Verification items for the finished model (mm, model axes). Round coordinates to 2 decimals unless told otherwise and drop trailing zeros. Loops run counter-clockwise (first coordinate to the right, second up) from the corner with the lowest first, then second, coordinate; pieces in that order, holes last. Notation, with made-up numbers: (1, 19.25) -> (22, 19.25) arc R16 ccw to (22, 33.25) -> close; hole circle Ø6 at (80, -36.75). An arc over 180 degrees is marked (long way). Write item = value, one per line.
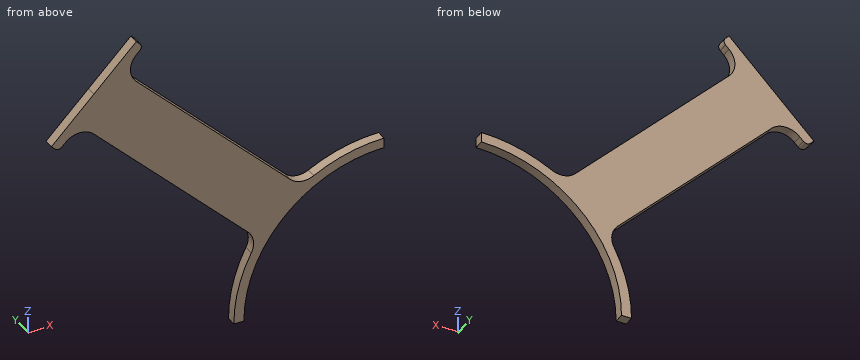
```python
from build123d import *

# Parameters (mm, degrees)
BOSS_EXTRUDE1_DEPTH = 5
FILLET1_R           = 10
FILLET2_R           = 2.5


with BuildPart() as part:
    # Sketch2 → Boss-Extrude1 (new body)
    with BuildSketch(Plane(origin=(0, 0, 0), x_dir=(1, 0, 0), z_dir=(0, 1, 0))):
        with BuildLine():
            Line((-70, 0), (-75, 0))
            ThreePointArc((-75, 0), (-53.033008589, -53.033008589), (0, -75))
            Line((0, -75), (0, -70))
            ThreePointArc((0, -70), (-49.497474683, -49.497474683), (-70, 0))
        make_face()
        with BuildLine():
            ThreePointArc((-41.354922509, -62.568125945), (-53.033008589, -53.033008589), (-62.568125945, -41.354922509))
            Line((-62.568125945, -41.354922509), (-152.027957955, -130.81475452))
            Line((-152.027957955, -130.81475452), (-162.634559673, -120.208152802))
            Line((-162.634559673, -120.208152802), (-166.170093579, -123.743686708))
            Line((-166.170093579, -123.743686708), (-144.956890143, -144.956890143))
            Line((-144.956890143, -144.956890143), (-123.743686708, -166.170093579))
            Line((-123.743686708, -166.170093579), (-120.208152802, -162.634559673))
            Line((-120.208152802, -162.634559673), (-130.81475452, -152.027957955))
            Line((-130.81475452, -152.027957955), (-41.354922509, -62.568125945))
        make_face()
    extrude(amount=BOSS_EXTRUDE1_DEPTH)

    # Fillet1
    fillet1_edges = [part.edges().sort_by_distance(p)[0] for p in [
        (-41.354922509, 2.5, 62.568125945),
        (-130.81475452, 2.5, 152.027957955),
        (-152.027957955, 2.5, 130.81475452),
        (-62.568125945, 2.5, 41.354922509),
    ]]
    fillet(fillet1_edges, radius=FILLET1_R)

    # Fillet2
    fillet2_edges = [part.edges().sort_by_distance(p)[0] for p in [
        (-120.208152802, 2.5, 162.634559673),
        (-162.634559673, 2.5, 120.208152802),
    ]]
    fillet(fillet2_edges, radius=FILLET2_R)


solid = part.part
```
(1) Sectioned sample at A-A, the plane y = 3. Record the cut outline in (x, z), and give its area (3 significant figures).
Filled sheet:
outline = (-166.17, 123.74) -> (-164.4, 121.98) arc R2.5 ccw to (-160.87, 121.98) -> (-159.1, 123.74) arc R10 cw to (-144.96, 123.74) -> (-68.05, 46.84) arc R10 cw to (-66.29, 35.09) arc R75 ccw to (-75, 0) -> (-70, 0) arc R70 cw to (0, 70) -> (0, 75) arc R75 ccw to (-35.09, 66.29) arc R10 cw to (-46.84, 68.05) -> (-123.74, 144.96) arc R10 cw to (-123.74, 159.1) -> (-121.98, 160.87) arc R2.5 ccw to (-121.98, 164.4) -> (-123.74, 166.17) -> close
area = 4,700 mm2
(2) Material ranges on probe 1 along Z at (x, y) = (-51, 1.45); probe 2 along Z at (x, y) = (-56.5, 1.3); probe 3 along X at (y, z) = (1.9, 63.5), recorded low to high. Write a range as from..to.
Filled sheet:
probe_1 = 47.95..72.21
probe_2 = 41.32..77.71
probe_3 = -84.71..-29.46
(3) Sectioned sample at C-C, the plane z = 135. Record the cut outline in (x, y).
Filled sheet:
outline = (-154.91, 0) -> (-113.79, 0) -> (-113.79, 5) -> (-154.91, 5) -> close
(4) Sectioned sample at B-B, the plane x = -142.5. Record the cut outline in (y, z).
Filled sheet:
outline = (0, 121.29) -> (5, 121.29) -> (5, 147.41) -> (0, 147.41) -> close
(5) Go/stop test with flat-tipped pins: pin 1 Ø3 at (y, z) = (1.5, 126.5) entering from -X; pin 2 Ø2 at (y, z) = (4, 27.5) entering from +X. Record where each tip stops, or that it passes through.
Filled sheet:
pin_1 = -164.91
pin_2 = -63.94
